Can you work these out from the model? Positions are in its coordinate system, mm. Face numbers are marked on the shaded views. A direction names the side the tool comes from. Give positions to 0.01 mm unless a question says otherwise; leave off trailing zeros. Order: outer loops, then holes, each group sorted by start corner. A loop starts at its lowest first (then second) coordinate and runs counter-clockwise, first axis right, second up. Notation, with made-up numbers: M 37,3 L 95,3 A33 ccw 95,41 Z; hole C 74.5,-10.75 d1. An arc over 180 degrees is marked long. Answer as a JSON object with one key per item and string values.
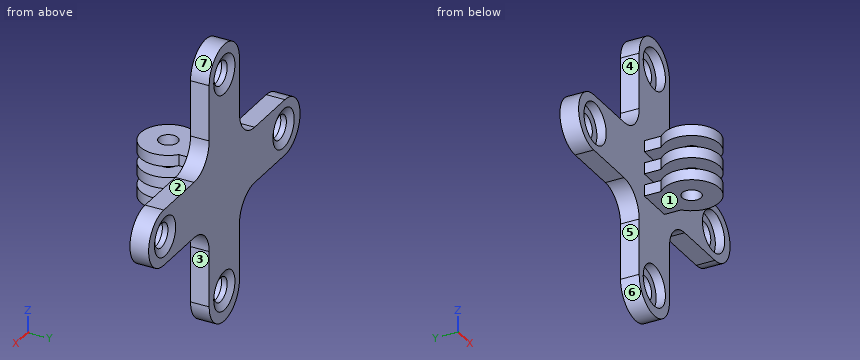
```python
from build123d import *

# Parameters (mm, degrees)
ESTRUSIONE_ESTRUSIONE1_DEPTH = 5
SCHIZZO4_R                   = 3.25
TAGLIO_ESTRUSIONE1_DEPTH     = 64.748958347
SMUSSO2_SIZE                 = 2
SMUSSO2_SIZE2                = 1
SCHIZZO5_R                   = 5.5
TAGLIO_ESTRUSIONE2_DEPTH     = 2.5
SCHIZZO7_R                   = 2.54
ESTRUSIONE_ESTRUSIONE2_DEPTH = 20
SCHIZZO9_W                   = 20
SCHIZZO9_H                   = 3
SCHIZZO9_H_2                 = 4.712842408
SCHIZZO9_H_3                 = 4.145579672
TAGLIO_ESTRUSIONE3_DEPTH     = 20


with BuildPart() as part:
    # Schizzo3 → Estrusione-Estrusione1 (new body)
    with BuildSketch(Plane(origin=(0, 0, 0), x_dir=(1, 0, 0), z_dir=(0, 1, 0))):
        with BuildLine():
            Line((-25.964231013, 18.101035176), (-10.964231013, 18.101035176))
            ThreePointArc((-10.964231013, 18.101035176), (-5.660930154, 20.297734317), (-3.464231013, 25.601035176))
            Line((-3.464231013, 25.601035176), (-3.464231013, 40.601035176))
            ThreePointArc((-3.464231013, 40.601035176), (4.035768987, 48.101035176), (11.535768987, 40.601035176))
            Line((11.535768987, 40.601035176), (11.535768987, 25.601035176))
            ThreePointArc((11.535768987, 25.601035176), (13.732468128, 20.297734317), (19.035768987, 18.101035176))
            Line((19.035768987, 18.101035176), (34.035768987, 18.101035176))
            ThreePointArc((34.035768987, 18.101035176), (41.535768987, 10.601035176), (34.035768987, 3.101035176))
            Line((34.035768987, 3.101035176), (19.035768987, 3.101035176))
            ThreePointArc((19.035768987, 3.101035176), (13.732468128, 0.904336035), (11.535768987, -4.398964824))
            Line((11.535768987, -4.398964824), (11.535768987, -19.398964824))
            ThreePointArc((11.535768987, -19.398964824), (4.035768987, -26.898964824), (-3.464231013, -19.398964824))
            Line((-3.464231013, -19.398964824), (-3.464231013, -4.398964824))
            ThreePointArc((-3.464231013, -4.398964824), (-5.660930154, 0.904336035), (-10.964231013, 3.101035176))
            Line((-10.964231013, 3.101035176), (-25.964231013, 3.101035176))
            ThreePointArc((-25.964231013, 3.101035176), (-33.464231013, 10.601035176), (-25.964231013, 18.101035176))
        make_face()
    extrude(amount=ESTRUSIONE_ESTRUSIONE1_DEPTH)

    # Schizzo4 → Taglio-Estrusione1 (cut, through all)
    with BuildSketch(Plane(origin=(0, 5, 0), x_dir=(1, 0, 0), z_dir=(0, 1, 0))):
        with Locations(Location((4.035768987, -18.733964824, 0), (0, 0, 270))):
            Circle(SCHIZZO4_R)
        with Locations(Location((4.035768987, 39.936035176, 0), (0, 0, 270))):
            Circle(SCHIZZO4_R)
        with Locations(Location((-25.299231013, 10.601035176, 0), (0, 0, 270))):
            Circle(SCHIZZO4_R)
        with Locations(Location((33.370768987, 10.601035176, 0), (0, 0, 270))):
            Circle(SCHIZZO4_R)
    extrude(amount=-TAGLIO_ESTRUSIONE1_DEPTH, mode=Mode.SUBTRACT)

    # Smusso2
    smusso2_edges = [part.edges().sort_by_distance(p)[0] for p in [
        (4.035768987, 5, 15.483964824),
        (4.035768987, 5, -43.186035176),
        (-25.299231013, 5, -13.851035176),
        (33.370768987, 5, -13.851035176),
    ]]
    smusso2_side = [part.faces().sort_by_distance(p)[0] for p in [
        (4.035768987, 5, -10.601035176),
    ]]
    chamfer(smusso2_edges, length=SMUSSO2_SIZE, length2=SMUSSO2_SIZE2, reference=smusso2_side[0])

    # Schizzo5 → Taglio-Estrusione2 (cut)
    with BuildSketch(Plane.XZ):
        with Locations(Location((4.03661079, 18.733616138, 0), (0, 0, 270))):
            Circle(SCHIZZO5_R)
        with Locations(Location((4.03661079, -39.936383862, 0), (0, 0, 270))):
            Circle(SCHIZZO5_R)
        with Locations(Location((-25.29838921, -10.601383862, 0), (0, 0, 270))):
            Circle(SCHIZZO5_R)
        with Locations(Location((33.370420301, -10.600193374, 0), (0, 0, 270))):
            Circle(SCHIZZO5_R)
    extrude(amount=-TAGLIO_ESTRUSIONE2_DEPTH, mode=Mode.SUBTRACT)

    # Schizzo7 → Estrusione-Estrusione2 (add)
    with BuildSketch(Plane.XY):
        with BuildLine():
            Line((-0.941517405, -4.504101529), (-0.941517405, 0))
            Line((-0.941517405, 0), (9.058482595, 0))
            Line((9.058482595, 0), (9.058482595, -4.504101529))
            ThreePointArc((9.058482595, -4.504101529), (4.058482595, -17.43), (-0.941517405, -4.504101529))
        make_face()
        with Locations((4.058482595, -10)):
            Circle(SCHIZZO7_R, mode=Mode.SUBTRACT)
    extrude(amount=-ESTRUSIONE_ESTRUSIONE2_DEPTH)

    # Schizzo9 → Taglio-Estrusione3 (cut)
    with BuildSketch(Plane.XZ):
        with Locations((4.109140738, -7.601035176)):
            Rectangle(SCHIZZO9_W, SCHIZZO9_H)
        with Locations((4.109140738, -13.601035176)):
            Rectangle(SCHIZZO9_W, SCHIZZO9_H)
        with Locations((4.109140738, -0.744613972)):
            Rectangle(SCHIZZO9_W, SCHIZZO9_H_2)
        with Locations((4.109140738, -20.173825012)):
            Rectangle(SCHIZZO9_W, SCHIZZO9_H_3)
    extrude(amount=TAGLIO_ESTRUSIONE3_DEPTH, mode=Mode.SUBTRACT)


solid = part.part
```
1) I want a section at B-B on y = -10. Write out the boundary of the cut face in (x, z).
Results found:
{"outline": "M -3.37,-18.1 L 1.52,-18.1 L 1.52,-15.1 L -3.37,-15.1 Z; M -3.37,-12.1 L 1.52,-12.1 L 1.52,-9.1 L -3.37,-9.1 Z; M -3.37,-6.1 L 1.52,-6.1 L 1.52,-3.1 L -3.37,-3.1 Z; M 6.6,-18.1 L 11.49,-18.1 L 11.49,-15.1 L 6.6,-15.1 Z; M 6.6,-12.1 L 11.49,-12.1 L 11.49,-9.1 L 6.6,-9.1 Z; M 6.6,-6.1 L 11.49,-6.1 L 11.49,-3.1 L 6.6,-3.1 Z"}
2) I need wall thicknesses on L1, parallel to Z at x = 0, y = -0.25; L2, parallel to Z at x = -12.5, y = 1.75; L3, parallel to X at y = -2.25, z = -5.5. Which ranges of each line are inside material? Lowest first, please.
Results found:
{"L1": "z = -18.1 to -15.1, -12.1 to -9.1, -6.1 to -3.1", "L2": "z = -18.1 to -3.1", "L3": "x = -0.94 to 9.06"}
3) Thinking about a two-plate mould opening in Z: for the marked faces 5, 6 and 7, which applies, pulls with the +Z half, pulls with the -Z half, needs draft (parallel to the pull), parting line crosses it, or undercut?
Results found:
{"face 5": "needs draft", "face 6": "pulls with the -Z half", "face 7": "pulls with the +Z half"}
4) For the marked faces 1, 2, 3 and 4, which set-ups out of +Z, -Z, +X, -X, +Y, -Y let a thin tool reach every point of the face, with its end or its side?
Results found:
{"face 1": "-Z, +X, -X, -Y", "face 2": "+Z, +X, +Y, -Y", "face 3": "-Z, +X, +Y, -Y", "face 4": "+Z, -X, +Y, -Y"}
5) I want a section at C-C on x = 20. Write out the boundary of the cut face in (y, z), and give its area (3 significant figures).
Results found:
{"outline": "M 0,-18.1 L 5,-18.1 L 5,-3.1 L 0,-3.1 Z", "area": "75.0 mm²"}
6) I want a section at D-D on z = 1. Write out the boundary of the cut face in (x, y).
Results found:
{"outline": "M -4.28,0 L 12.35,0 L 12.35,5 L -4.28,5 Z"}
7) I'm going to push flat-ended pins straight in: pin 1 Ø17.5 at (x, z) = (4.04, 18.73) entering from +Y; pin 2 Ø5.5 at (x, z) = (6.5, -42) entering from -Y; pin 3 Ø8 at (x, y) = (-5, -5.5) entering from -Z; pin 4 Ø1.5 at (y, z) = (-2.5, -16) entering from -X. Where does each tip first touch, or does it pass through?
Results found:
{"pin 1": "stops at y = 5", "pin 2": "stops at y = 0", "pin 3": "stops at z = -18.1", "pin 4": "stops at x = -0.94"}
8) I want a section at A-A on y = -2.5. Write out the boundary of the cut face in (x, z), and give its area (3 significant figures).
Results found:
{"outline": "M -0.94,-18.1 L 9.06,-18.1 L 9.06,-15.1 L -0.94,-15.1 Z; M -0.94,-12.1 L 9.06,-12.1 L 9.06,-9.1 L -0.94,-9.1 Z; M -0.94,-6.1 L 9.06,-6.1 L 9.06,-3.1 L -0.94,-3.1 Z", "area": "90.0 mm²"}
